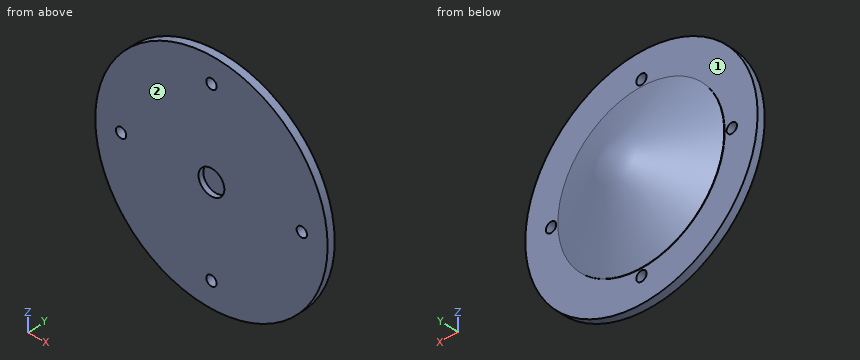
Autodesk Inventor part; units mm, degrees
ref_plane "YZ Plane" through (0, 0, 0) normal (1, 0, 0) x (0, 1, 0)
ref_plane "XZ Plane" through (0, 0, 0) normal (0, 1, 0) x (-1, 0, 0)
ref_plane "XY Plane" through (0, 0, 0) normal (0, 0, 1) x (1, 0, 0)
sketch "Szkic1" plane through (0, 0, 0) normal (0, 1, 0) x (-1, 0, 0)
  circle A0 centre (0, 0) radius 45
  circle A1 centre (35, 0) radius 1.5
  circle A2 centre (-35, 0) radius 1.5
  circle A3 centre (0, 35) radius 1.5
  circle A4 centre (0, -35) radius 1.5
  dimension "d0" = 90
  dimension "d30" = 3
  dimension "d31" = 3
  dimension "d32" = 3
  dimension "d33" = 3
extrude "Wyciągnięcie proste1" add sketch "Szkic1" along normal blind 3 contours A0 | A1 | A2 | A3 | A4
sketch "Szkic4" plane through (0, 0, 0) normal (0, -1, 0) x (1, 0, 0)
  circle A0 centre (0, 0) radius 2.5
  circle A1 centre (0, 0) radius 5
  dimension "d19" = 10
extrude "Wyciągnięcie proste5" cut sketch "Szkic4" against normal blind 2 contours A0 | A1
sketch "Szkic8" plane through (0, 2, 0) normal (0, -1, 0) x (1, 0, 0)
  point P0 (0, 0)
sketch "Szkic17" plane through (0, 3, 0) normal (0, 1, 0) x (1, 0, 0)
  circle A0 centre (-35, 0) radius 2
  circle A1 centre (0, 35) radius 2
  circle A2 centre (0, -35) radius 2
  circle A3 centre (35, 0) radius 2
  point P0 (0, 0)
  dimension "d34" = 4
  dimension "d35" = 4
  dimension "d36" = 4
  dimension "d37" = 4
extrude "Wyciągnięcie proste9" cut sketch "Szkic17" against normal blind 47
sketch "Szkic19" plane through (0, 3, 0) normal (0, 1, 0) x (1, 0, 0)
  point P0 (0, 0)
sketch "Szkic20" plane through (0, 3, 0) normal (0, 1, 0) x (1, 0, 0)
  circle A0 centre (0, 0) radius 5
  circle A1 centre (0, 0) radius 32.25
  dimension "d47" = 64.5
extrude "Wyciągnięcie proste11" add sketch "Szkic20" along normal blind 15 contours A0 | A1
chamfer "Faza1" distance 32.25 angle 24.7 1 edges at (-32.25, 18, 0) measured on face at (15.449, 18, -8.9531)
properties part number "tarcza"
Read the model definition and answer for the solid it produces. Units are mm, in the model's axes. Face numbers are marked on the shaded views. A direction names the side the tool comes from. Round coordinates to 2 decimals unless told otherwise and drop trailing zeros. Write each loop counter-clockwise with the first axis right and the second up, starting at its lowest first coordinate (ties: lowest second). Pieces come first, ordered by that corner, then holes. Notation, with made-up numbers: (54.25, 49.5) - (95.25, 49.5) arc R20 cw to (95.25, 68.5) - close; hole circle Ø7 at (61, 87.25). An arc over 180 degrees is marked (long way). One line per question, with ' | ' between items. Start each with the question number.
1. Section A-A (x = -35) is taken. Determine the outline of the cut face in (y, z).
2. Section B-B (z = -35) is taken. Determine the outline of the cut face in (x, y).
3. Each of these flat-tipped pins is pushed along its axis until it touches: pin 1 (12 mm diameter, centred on x = 1.5, z = 19.5, fed in from +Y); pin 2 (6 mm diameter, centred on x = 14.5, y = 6.5, fed in from +Z); pin 3 (4 mm diameter, centred on x = 30, z = 16, fed in from +Y); pin 4 (8 mm diameter, centred on x = 0.5, z = 1, fed in from -Y). Where does it stop, or does it pass through?
4. Find the intervals of material crossed by probe 1 along Z at (x, y) = (0, 0.9); probe 2 along Z at (x, y) = (0, 2.4); probe 3 along X at (y, z) = (2.15, 35), in increasing order. Write a range as [from, to].
5. Section C-C (y = 14.5) is taken. Determine the outline of the cut face in (x, z).
6. For the marked faces 1 and 2, determine the directions among +Z, -Z, +X, -X, +Y, -Y from which every point of the face is accessible in a straight line to the end or side of a thin tool.
Filled in:
1) outline: (0, -28.28) - (3, -28.28) - (3, -2) - (0, -2) - close; (0, 2) - (3, 2) - (3, 28.28) - (0, 28.28) - close
2) outline: (-28.28, 0) - (-2, 0) - (-2, 3) - (-28.28, 3) - close; (2, 0) - (28.28, 0) - (28.28, 3) - (2, 3) - close
3) pin 1: y = 11.76 | pin 2: z = 28.15 | pin 3: y = 3.28 | pin 4: y = 0
4) probe 1: [-45, -37], [-33, -5], [5, 33], [37, 45] | probe 2: [-45, -37], [-33, 33], [37, 45] | probe 3: [-28.28, -2], [2, 28.28]
5) outline: circle Ø15.22 at (0, 0)
6) face 1: +Y | face 2: +Z, -Z, +X, -X, -Y
